Part model, mm, in its own coordinate system. A direction names the side the tool comes from. Round coordinates to 2 decimals unless told otherwise and drop trailing zeros. Write each loop counter-clockwise with the first axis right and the second up, starting at its lowest first coordinate (ties: lowest second). Pieces come first, ordered by that corner, then holes. Notation, with made-up numbers: M 85.25,-1.75 L 90.25,-1.75 A14 cw 90.25,3.25 Z; hole C 8.25,34 d7. An arc over 180 degrees is marked long. Answer as a JSON object with one key per item and string values. Group by question number.
1. Band-saw the part on A-A, the plane z = 2.5. Write the cut outline in (x, y).
2. Drill centre lines: line 1 (X direction, y = -14, z = 0.7); line 2 (Z direction, x = -2, y = 0); line 3 (Y direction, x = -3.5, z = 3.25). Where is each one in solid material? Low to high. Write a range as from..to.
3. Which spindle directions (+Z, -Z, +X, -X, +Y, -Y) get a long thin tool onto all of the face, cutting with end or side? Do faces 4 (the face through (3, -12.3, 3.5)), 5 (the face through (0, 0, 26)). Say none if no direction does.
4. Drop flat-ended pins along their axis: pin 1 (6 mm diameter, centred on x = 0, y = 14, fed in from +Z); pin 2 (4 mm diameter, centred on x = 0.5, z = 13, fed in from +Y); pin 3 (7.5 mm diameter, centred on y = 0, z = 18, fed in from +X); pin 4 (7.5 mm diameter, centred on x = 0.5, y = -15, fed in from +Z). Give the stop position or say it passes through.
5. Band-saw the part on B-B, the plane x = -6. Write the cut outline in (y, z), plus the area to 3 significant figures.
6. Band-saw the part on C-C, the plane y = 3. Write the cut outline in (x, z), plus the area to 3 significant figures.
7. Two-plate mould, pull along Y, no slides. Class faces 1 (the face through (3, -15.7, 3.5)), 2 (the face through (3.4, -12.6, 5)), 3 (the face through (0, 8, 11)): +Y half, -Y half, draft (parallel to the pull), parting line (faces both ways), or undercut.
8. Band-saw the part on D-D, the plane z = 15.25. Write the cut outline in (x, y).
from build123d import *

# Parameters (mm, degrees)
SKETCH_R        = 4.05
PAD_DEPTH       = 7.5
POCKET_DEPTH    = 3.1
SKETCH002_R     = 2.5
POCKET001_DEPTH = 126.020998


with BuildPart() as part:
    # Sketch → Pad (new body, symmetric)
    with BuildSketch(Plane.YZ):
        with BuildLine():
            Line((-20, 0), (20, 0))
            Line((20, 0), (20, 5))
            Line((20, 5), (8, 5))
            Line((8, 5), (8, 18))
            ThreePointArc((8, 18), (0, 26), (-8, 18))
            Line((-8, 18), (-8, 5))
            Line((-8, 5), (-20, 5))
            Line((-20, 5), (-20, 0))
        make_face()
        with Locations((0, 18)):
            Circle(SKETCH_R, mode=Mode.SUBTRACT)
    extrude(amount=PAD_DEPTH, both=True)

    # Sketch001 (on Face7 of Pad) → Pocket (cut)
    with BuildSketch(Plane(origin=(0, 0, 5), x_dir=(0, -1, 0), z_dir=(0, 0, 1))):
        Polygon((-10.55, 1.991858), (-14, 3.983717), (-17.45, 1.991858), (-17.45, -1.991858), (-14, -3.983717), (-10.55, -1.991858), align=None)
    pocket = extrude(amount=-POCKET_DEPTH, mode=Mode.SUBTRACT)

    # Sketch002 (on Face1 of Pocket) → Pocket001 (cut, through all)
    with BuildSketch(Plane.YX):
        with Locations((14, 0)):
            Circle(SKETCH002_R)
    pocket001 = extrude(amount=-POCKET001_DEPTH, mode=Mode.SUBTRACT)

    # Mirrored: Pocket, Pocket001 across XZ
    add(pocket.mirror(Plane.XZ), mode=Mode.SUBTRACT)
    add(pocket001.mirror(Plane.XZ), mode=Mode.SUBTRACT)


solid = part.part
Worked answers:
{
 "1": {"outline": "M -7.5,-20 L 7.5,-20 L 7.5,20 L -7.5,20 Z; hole M -3.98,-14 L -1.99,-17.45 L 1.99,-17.45 L 3.98,-14 L 1.99,-10.55 L -1.99,-10.55 Z; hole M -3.98,14 L -1.99,10.55 L 1.99,10.55 L 3.98,14 L 1.99,17.45 L -1.99,17.45 Z"},
 "2": {"line 1": "x = -7.5..-2.5, 2.5..7.5", "line 2": "z = 0..13.95, 22.05..26", "line 3": "y = -20..-14.84, -13.16..13.16, 14.84..20"},
 "3": {"face 4": "+Z", "face 5": "+Z, +X, -X"},
 "4": {"pin 1": "stops at z = 1.9", "pin 2": "stops at y = 8", "pin 3": "passes through", "pin 4": "stops at z = 5"},
 "5": {"outline": "M -20,0 L 20,0 L 20,5 L 8,5 L 8,18 A8 ccw -8,18 L -8,5 L -20,5 Z; hole C 0,18 d8.1", "area": "457 mm^2"},
 "6": {"outline": "M -7.5,0 L 7.5,0 L 7.5,15.28 L -7.5,15.28 Z; M -7.5,20.72 L 7.5,20.72 L 7.5,25.42 L -7.5,25.42 Z", "area": "300 mm^2"},
 "7": {"face 1": "undercut", "face 2": "draft", "face 3": "+Y half"},
 "8": {"outline": "M -7.5,-8 L 7.5,-8 L 7.5,-2.97 L -7.5,-2.97 Z; M -7.5,2.97 L 7.5,2.97 L 7.5,8 L -7.5,8 Z"}
}
